```python
from build123d import *

# Parameters (mm, degrees)
SKETCH1_W           = 37.5
SKETCH1_H           = 65.4
BOSS_EXTRUDE1_DEPTH = 9.15
FILLET1_R           = 9.15


with BuildPart() as part:
    # Sketch1 → Boss-Extrude1 (new, symmetric)
    with BuildSketch(Plane(origin=(0, 0, 0), x_dir=(1, 0, 0), z_dir=(0, 1, 0))):
        Rectangle(SKETCH1_W, SKETCH1_H)
    extrude(amount=BOSS_EXTRUDE1_DEPTH, both=True)

    # Fillet1
    fillet1_edges = [part.edges().sort_by_distance(p)[0] for p in [
        (18.75, -9.15, 0),
        (18.75, 9.15, 0),
        (-18.75, -9.15, 0),
        (-18.75, 9.15, 0),
    ]]
    fillet(fillet1_edges, radius=FILLET1_R - 0.0001)  # a hair under: the kernel refuses the full size


solid = part.part
```
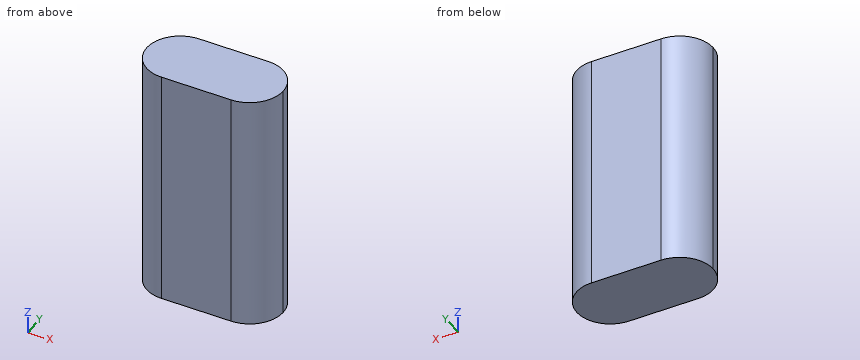
Design review of the part built by this model. Coordinates are the model's own, in mm. Give positions to 0.01 mm unless a question says otherwise; leave off trailing zeros. Loops run counter-clockwise (first coordinate to the right, second up) from the corner with the lowest first, then second, coordinate; pieces in that order, holes last. Notation, with made-up numbers: (-3.75, 36.5) -> (51.25, 36.5) arc R15 ccw to (51.25, 44.5) -> close; hole circle Ø4 at (27.5, -9.5). An arc over 180 degrees is marked (long way). One line per item, written item: value.
Q1. We need section B-B on y = -4.5. Give the boundary of the cut face in (x, z).
Numbers:
outline: (-17.57, -32.7) -> (17.57, -32.7) -> (17.57, 32.7) -> (-17.57, 32.7) -> close
Q2. We need section C-C on x = -13.5. Give the boundary of the cut face in (y, z).
Numbers:
outline: (-8.28, -32.7) -> (8.28, -32.7) -> (8.28, 32.7) -> (-8.28, 32.7) -> close
Q3. For L1, parallel to X at y = -1.75, z = -5.5; L2, parallel to Y at x = 10, z = -23; L3, parallel to X at y = 4.25, z = -11.5, list the stretches that pass through material, from the lowest coordinate up.
Numbers:
L1: x = -18.58 to 18.58
L2: y = -9.14 to 9.14
L3: x = -17.7 to 17.7
